```python
from build123d import *

# Parameters (mm, degrees)
SKETCH1_R           = 1.1
BOSS_EXTRUDE1_DEPTH = 0.75
SKETCH2_R           = 1.55
SKETCH2_R_2         = 1.1
BOSS_EXTRUDE2_DEPTH = 4


with BuildPart() as part:
    # Sketch1 → Boss-Extrude1 (new body)
    with BuildSketch(Plane(origin=(0, 0, 0), x_dir=(1, 0, 0), z_dir=(0, 1, 0))):
        with BuildLine():
            Line((11, -3.99967418), (11, 3))
            Line((11, 3), (3, 3))
            Line((3, 3), (3, 11))
            Line((3, 11), (-3.99967418, 11))
            Line((-3.99967418, 11), (-3.99967418, 0))
            ThreePointArc((-3.99967418, 0), (-2.828196736, -2.828196736), (0, -3.99967418))
            Line((0, -3.99967418), (11, -3.99967418))
        make_face()
        with Locations(Location((0, 0, 0), (0, 0, 270))):
            Circle(SKETCH1_R, mode=Mode.SUBTRACT)
    extrude(amount=BOSS_EXTRUDE1_DEPTH)

    # Sketch2 → Boss-Extrude2 (add)
    with BuildSketch(Plane(origin=(0, 0.75, 0), x_dir=(1, 0, 0), z_dir=(0, 1, 0))):
        with Locations(Location((0, 0, 0), (0, 0, 270))):
            Circle(SKETCH2_R)
        with Locations(Location((0, 0, 0), (0, 0, 270))):
            Circle(SKETCH2_R_2, mode=Mode.SUBTRACT)
    extrude(amount=BOSS_EXTRUDE2_DEPTH)


solid = part.part
```
Model file for the job. Use its own axes, mm. Give positions to 0.01 mm unless a question says otherwise; leave off trailing zeros. Loops run counter-clockwise (first coordinate to the right, second up) from the corner with the lowest first, then second, coordinate; pieces in that order, holes last. Notation, with made-up numbers: (25, -3) - (34, -3) arc R16 cw to (34, 28) - close; hole circle Ø9 at (64, 81). An arc over 180 degrees is marked (long way). One line per item, written item: value. Start each with the question number.
1. Slice it at C-C (x = 8.5). List the corners of the cut face in (y, z), plus the area to 3 significant figures.
2. Probe L1, parallel to X at y = 3.5, z = 0; L2, parallel to Y at x = 2.25, z = -6.5; L3, parallel to X at y = 2.7, z = -1.25. List the from-to ranges inside material, lowest first. Write a range as from..to.
3. Slice it at B-B (y = 2.2). List the corners of the cut face in (x, z).
4. Pin check, flat tips, straight feed: pin 1 (3 mm diameter, centred on x = 1.5, z = -4, fed in from +Y); pin 2 (0.6 mm diameter, centred on x = 5, y = 0, fed in from -Z); pin 3 (0.8 mm diameter, centred on y = 0.5, z = -6.5, fed in from +X). Stop position of each tip, or through.
5. Pull direction X, two halves, no side cores. Call faces 1 (the cylindrical face through (-2.859, 0.37, 2.797)), 2 (the cylindrical face through (0.466, 2.722, 1.478)), 3 (the cylindrical face through (1.09, 2.34, -0.14)): pulls with the +X half, pulls with the -X half, needs draft (parallel to the pull), parting line crosses it, or undercut.
6. Slice it at A-A (x = -0.25). List the corners of the cut face in (y, z).
7. Slice it at D-D (z = -8). List the corners of the cut face in (x, y), plus the area to 3 significant figures.
Solution:
1. outline: (0, -3) - (0.75, -3) - (0.75, 4) - (0, 4) - close
1. area: 5.25 mm^2
2. L1: x = -1.55..-1.1, 1.1..1.55
2. L2: y = 0..0.75
2. L3: x = -0.92..0.92
3. outline: circle Ø3.1 at (0, 0); hole circle Ø2.2 at (0, 0)
4. pin 1: stops at y = 0.75
4. pin 2: stops at z = -3
4. pin 3: stops at x = 3
5. face 1: pulls with the -X half
5. face 2: parting line crosses it
5. face 3: undercut
6. outline: (0, -11) - (0.75, -11) - (0.75, -1.53) - (4.75, -1.53) - (4.75, -1.07) - (0, -1.07) - close; (0, 1.07) - (4.75, 1.07) - (4.75, 1.53) - (0.75, 1.53) - (0.75, 3.99) - (0, 3.99) - close
7. outline: (-4, 0) - (3, 0) - (3, 0.75) - (-4, 0.75) - close
7. area: 5.25 mm^2
